Input: part model. Units: mm. Frame: model coordinates. A direction names the side the tool comes from. Round coordinates to 2 decimals unless told otherwise and drop trailing zeros. Loops run counter-clockwise (first coordinate to the right, second up) from the corner with the lowest first, then second, coordinate; pieces in that order, holes last. Notation, with made-up numbers: M 48,53 L 62,53 A22 ccw 62,82 Z; hole C -37.75,-18 d11. An arc over 180 degrees is marked long. Put each result on its own line as item: value. Start each with the question number.
1) Reachability of faces 1 (the face through (-9.64, 5.51, -1.23)), 2 (the face through (-13, 0, 0)) from +Z, -Z, +X, -X, +Y, -Y: full face, straight path, thin tool, end or side. Return the list, or none.
2) Section D-D on y = -9.5. Output: boundary loops of the cut face in (x, z).
3) Pin query (flat end, axial travel): pin 1 (2 mm diameter, centred on x = 9, y = 20, fed in from -Z); pin 2 (5 mm diameter, centred on x = -5.5, y = -7.5, fed in from -Z); pin 3 (1.2 mm diameter, centred on x = -10, z = -1.5, fed in from -Y); pin 4 (1.5 mm diameter, centred on x = -7.5, y = 6, fed in from -Z). Return the tip coordinate at first contact, or that it passes through.
4) Section B-B on x = -1. Output: boundary loops of the cut face in (y, z).
5) Line query: probe 1 along Y at (x, z) = (9, 2.15); probe 2 along Y at (x, z) = (7, 0.4); probe 3 along Y at (x, z) = (9, 1.65). Output: solid intervals per line, ascending.
6) Section C-C on y = 0. Output: boundary loops of the cut face in (x, z), plus the area to 3 significant figures.
7) Draft query along X for faces 3 (the face through (13, 0, 0)), 4 (the face through (1, -10.5, 3)), 5 (the face through (-6.36, 21.49, -1.23)). Return one class per face: +X half, -X half, draft (parallel to the pull), parting line (faces both ways), or undercut.
8) Section A-A on z = 0.9. State how many separate pieces and enclosed holes the cut face has, plus the area to 3 significant figures.
from build123d import *

# Parameters (mm, degrees)
F0_R     = 1.75
F1_DEPTH = 2
F3_DEPTH = 2.5
F4_R     = 1.75
F5_DEPTH = 1.5


with BuildPart() as f1:
    # F0 (on Top) → F1 (new body)
    with BuildSketch(Plane.XY):
        with BuildLine():
            ThreePointArc((-9, -24), (-6.171573, -22.828427), (-5, -20))
            ThreePointArc((-5, -20), (-9, -16), (-13, -20))
            ThreePointArc((-13, -20), (-11.828427, -22.828427), (-9, -24))
        make_face()
        with Locations((-9, -20)):
            Circle(F0_R, mode=Mode.SUBTRACT)
        with BuildLine():
            ThreePointArc((-13, -20), (-9, -16), (-5, -20))
            ThreePointArc((-5, -20), (-6.171573, -22.828427), (-9, -24))
            Line((-9, -24), (9, -24))
            ThreePointArc((9, -24), (6.171573, -17.171573), (13, -20))
            Line((13, -20), (13, 20))
            ThreePointArc((13, 20), (6.171573, 17.171573), (9, 24))
            Line((9, 24), (-9, 24))
            ThreePointArc((-9, 24), (-6.171573, 22.828427), (-5, 20))
            ThreePointArc((-5, 20), (-9, 16), (-13, 20))
            Line((-13, 20), (-13, -20))
        make_face()
        with Locations((-7, -7)):
            Circle(F0_R, mode=Mode.SUBTRACT)
        with Locations((7, -7)):
            Circle(F0_R, mode=Mode.SUBTRACT)
        with Locations((-7, 7)):
            Circle(F0_R, mode=Mode.SUBTRACT)
        with Locations((7, 7)):
            Circle(F0_R, mode=Mode.SUBTRACT)
        with BuildLine():
            ThreePointArc((-9, 24), (-11.828427, 22.828427), (-13, 20))
            ThreePointArc((-13, 20), (-9, 16), (-5, 20))
            ThreePointArc((-5, 20), (-6.171573, 22.828427), (-9, 24))
        make_face()
        with Locations((-9, 20)):
            Circle(F0_R, mode=Mode.SUBTRACT)
        with BuildLine():
            ThreePointArc((13, -20), (6.171573, -17.171573), (9, -24))
            ThreePointArc((9, -24), (11.828427, -22.828427), (13, -20))
        make_face()
        with Locations((9, -20)):
            Circle(F0_R, mode=Mode.SUBTRACT)
        with BuildLine():
            ThreePointArc((13, 20), (11.828427, 22.828427), (9, 24))
            ThreePointArc((9, 24), (6.171573, 17.171573), (13, 20))
        make_face()
        with Locations((9, 20)):
            Circle(F0_R, mode=Mode.SUBTRACT)
    extrude(amount=F1_DEPTH)

    # F2 (on face) → F3 (join)
    with BuildSketch(Plane(origin=(0, 0, 0), x_dir=(1, 0, 0), z_dir=(0, 0, -1))):
        with BuildLine():
            ThreePointArc((-9, 24), (-11.828427, 22.828427), (-13, 20))
            Line((-13, 20), (-13, -20))
            ThreePointArc((-13, -20), (-11.828427, -22.828427), (-9, -24))
            Line((-9, -24), (9, -24))
            ThreePointArc((9, -24), (11.828427, -22.828427), (13, -20))
            Line((13, -20), (13, 20))
            ThreePointArc((13, 20), (11.828427, 22.828427), (9, 24))
            Line((9, 24), (-9, 24))
        make_face()
        Polygon((-7.25, -16.968911), (-5.5, -20), (-7.25, -23.031089), (-10.75, -23.031089), (-12.5, -20), (-10.75, -16.968911), align=None, mode=Mode.SUBTRACT)
        Polygon((-5.25, -3.968911), (-3.5, -7), (-5.25, -10.031089), (-8.75, -10.031089), (-10.5, -7), (-8.75, -3.968911), align=None, mode=Mode.SUBTRACT)
        Polygon((10.75, -16.968911), (12.5, -20), (10.75, -23.031089), (7.25, -23.031089), (5.5, -20), (7.25, -16.968911), align=None, mode=Mode.SUBTRACT)
        Polygon((8.75, -3.968911), (10.5, -7), (8.75, -10.031089), (5.25, -10.031089), (3.5, -7), (5.25, -3.968911), align=None, mode=Mode.SUBTRACT)
        Polygon((-8.75, 10.031089), (-5.25, 10.031089), (-3.5, 7), (-5.25, 3.968911), (-8.75, 3.968911), (-10.5, 7), align=None, mode=Mode.SUBTRACT)
        Polygon((-7.25, 23.031089), (-5.5, 20), (-7.25, 16.968911), (-10.75, 16.968911), (-12.5, 20), (-10.75, 23.031089), align=None, mode=Mode.SUBTRACT)
        Polygon((8.75, 10.031089), (10.5, 7), (8.75, 3.968911), (5.25, 3.968911), (3.5, 7), (5.25, 10.031089), align=None, mode=Mode.SUBTRACT)
        Polygon((7.25, 23.031089), (10.75, 23.031089), (12.5, 20), (10.75, 16.968911), (7.25, 16.968911), (5.5, 20), align=None, mode=Mode.SUBTRACT)
    extrude(amount=F3_DEPTH)

    # F4 (on face) → F5 (join)
    with BuildSketch(Plane.XY.offset(2)):
        with BuildLine():
            Line((-10.5, 10.5), (10.5, 10.5))
            Line((10.5, 10.5), (13, 10.5))
            Line((13, 10.5), (13, 20))
            ThreePointArc((13, 20), (11.828427, 22.828427), (9, 24))
            Line((9, 24), (-9, 24))
            ThreePointArc((-9, 24), (-11.828427, 22.828427), (-13, 20))
            Line((-13, 20), (-13, -20))
            ThreePointArc((-13, -20), (-11.828427, -22.828427), (-9, -24))
            Line((-9, -24), (9, -24))
            ThreePointArc((9, -24), (11.828427, -22.828427), (13, -20))
            Line((13, -20), (13, -10.5))
            Line((13, -10.5), (10.5, -10.5))
            Line((10.5, -10.5), (-10.5, -10.5))
            Line((-10.5, -10.5), (-10.5, 10.5))
        make_face()
        with Locations((-9, -20)):
            Circle(F4_R, mode=Mode.SUBTRACT)
        with Locations((9, -20)):
            Circle(F4_R, mode=Mode.SUBTRACT)
        with Locations((-9, 20)):
            Circle(F4_R, mode=Mode.SUBTRACT)
        with Locations((9, 20)):
            Circle(F4_R, mode=Mode.SUBTRACT)
    extrude(amount=F5_DEPTH)


solid = f1.part
Geometry results:
1. face 1: -Z
1. face 2: +Z, -Z, -X, +Y, -Y
2. outline: M -13,-2.5 L -9.06,-2.5 L -9.06,0 L -4.94,0 L -4.94,-2.5 L 4.94,-2.5 L 4.94,0 L 9.06,0 L 9.06,-2.5 L 13,-2.5 L 13,2 L -10.5,2 L -10.5,3.5 L -13,3.5 Z
3. pin 1: passes through
3. pin 2: stops at z = -2.5
3. pin 3: stops at y = -23.98
3. pin 4: stops at z = 0
4. outline: M -24,-2.5 L 24,-2.5 L 24,3.5 L 10.5,3.5 L 10.5,2 L -10.5,2 L -10.5,3.5 L -24,3.5 Z
5. probe 1: y = -24 to -21.75, -18.25 to -10.5, 10.5 to 18.25, 21.75 to 24
5. probe 2: y = -24 to -8.75, -5.25 to 5.25, 8.75 to 24
5. probe 3: y = -24 to -21.75, -18.25 to 18.25, 21.75 to 24
6. outline: M -13,-2.5 L 13,-2.5 L 13,2 L -10.5,2 L -10.5,3.5 L -13,3.5 Z
6. area: 121 mm²
7. face 3: +X half
7. face 4: draft
7. face 5: undercut
8. separate pieces: 1
8. enclosed holes: 8
8. area: 1,160 mm²
